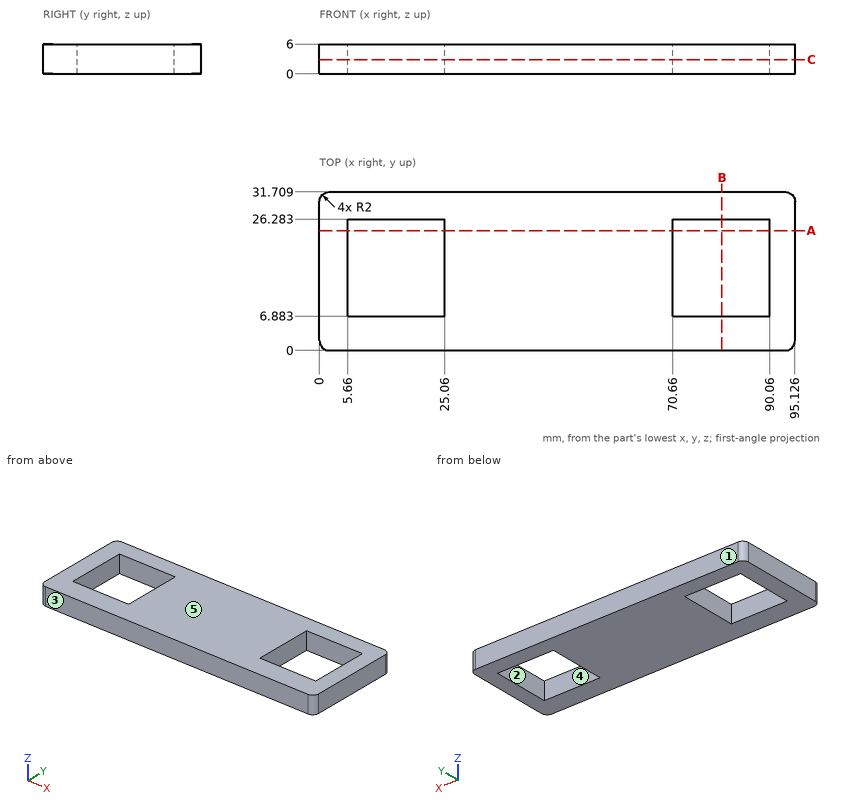
Print and shaded views of the part. All mm, measured from the part's lowest x, y and z. A direction names the side the tool comes from. Coordinates: 2 decimals unless noted, no trailing zeros. Write each loop counter-clockwise with the first axis right and the second up, starting at its lowest first coordinate (ties: lowest second). Pieces come first, ordered by that corner, then holes.
(1) 3-axis set-ups, long thin cutter, end or side, ignore diameter. For the marked faces 4 and 5: which of +Z, -Z, +X, -X, +Y, -Y reach the whole face in a straight line?
(2) Cut at C-C, the plane z = 2.85. List the corners of the cut face in (x, y), and give its area (3 significant figures).
(3) Two-plate mould, pull along Y, no slides. Class the marked faces 1, 2 and 3: +Y half, -Y half, draft (parallel to the pull), parting line (faces both ways), or undercut.
(4) Flat gauge pin, fed straight in: pin 1 (4 mm diameter, centred on x = 80.5, y = 4.5, fed in from -Z). Where does the tip first touch, or does it go through?
(5) Cut at B-B, the plane x = 80.5. List the corners of the cut face in (y, z).
(6) Drill centre lines: probe 1 along X at (y, z) = (7, 5.7); probe 2 along Y at (x, z) = (12.5, 0.75). Where is each one in solid material? Low to high.
(7) Cut at A-A, the plane y = 24. List the corners of the cut face in (x, z).
Geometry says:
1. face 4: +Z, -Z
1. face 5: +Z, +X, -X, +Y, -Y
2. outline: (0, 2) arc R2 ccw to (2, 0) - (93.13, 0) arc R2 ccw to (95.13, 2) - (95.13, 29.71) arc R2 ccw to (93.13, 31.71) - (2, 31.71) arc R2 ccw to (0, 29.71) - close; hole (5.66, 6.88) - (25.06, 6.88) - (25.06, 26.28) - (5.66, 26.28) - close; hole (70.66, 6.88) - (90.06, 6.88) - (90.06, 26.28) - (70.66, 26.28) - close
2. area: 2,260 mm2
3. face 1: +Y half
3. face 2: undercut
3. face 3: -Y half
4. pin 1: stops at z = 0
5. outline: (0, 0) - (6.88, 0) - (6.88, 6) - (0, 6) - close; (26.28, 0) - (31.71, 0) - (31.71, 6) - (26.28, 6) - close
6. probe 1: x = 0 to 5.66, 25.06 to 70.66, 90.06 to 95.13
6. probe 2: y = 0 to 6.88, 26.28 to 31.71
7. outline: (0, 0) - (5.66, 0) - (5.66, 6) - (0, 6) - close; (25.06, 0) - (70.66, 0) - (70.66, 6) - (25.06, 6) - close; (90.06, 0) - (95.13, 0) - (95.13, 6) - (90.06, 6) - close
